Verification items for the finished model (mm, model axes). A direction names the side the tool comes from. Give positions to 0.01 mm unless a question says otherwise; leave off trailing zeros. Loops run counter-clockwise (first coordinate to the right, second up) from the corner with the lowest first, then second, coordinate; pieces in that order, holes last. Notation, with made-up numbers: (11.25, 66) - (66.25, 66) arc R21 ccw to (66.25, 80) - close; hole circle Ø3 at (-17, 37). An arc over 180 degrees is marked (long way). Answer in a Markdown table with one row per item.
Autodesk Fusion 360 part; units mm, degrees
sketch "Sketch1" plane through (0, 0, 0) normal (0, 0, 1) x (1, 0, 0)
  line L0 (-3.85, 0) -> (3.85, 0) construction
  line L1 (-3.85, 0) -> (-8.35, 0) construction
  line L2 (3.85, 0) -> (8.35, 0) construction
  line L3 (0, 0) -> (0, -3.2) construction
  line L4 (-3.85, -4.5) -> (3.85, -4.5)
  line L5 (3.85, 4.5) -> (-3.85, 4.5)
  arc A0 (-3.85, 4.5) -> (-3.85, -4.5) centre (-3.85, 0) ccw
  arc A1 (3.85, -4.5) -> (3.85, 4.5) centre (3.85, 0) ccw
  line L6 (-0.9465, -2.8772) -> (-1.5, -4.5)
  line L7 (0.9465, -2.8772) -> (1.5, -4.5)
  arc A2 (0.9465, -2.8772) -> (-0.9465, -2.8772) centre (0, -3.2) ccw
  line L8 (11.5, -6) -> (-11.5, -6)
  line L9 (-11.5, -6) -> (-11.5, 6)
  line L10 (-11.5, 6) -> (11.5, 6)
  line L11 (11.5, 6) -> (11.5, -6)
  line L12 (11.5, -6) -> (-11.5, 6) construction
  line L13 (-11.5, -6) -> (11.5, 6) construction
  line L14 (-1.15, 2.75) -> (1.15, 2.75)
  line L15 (1.15, -0.75) -> (-1.15, -0.75)
  arc A3 (1.15, -0.75) -> (1.15, 2.75) centre (1.15, 1) ccw
  arc A4 (-1.15, 2.75) -> (-1.15, -0.75) centre (-1.15, 1) ccw
  line L16 (-1.15, 1) -> (1.15, 1)
  dimension "d1" = 9
  dimension "d2" = 16.7
  dimension "d3" = 2
  dimension "d4" = 3.2
  dimension "d5" = 3
  dimension "d6" = 12
  dimension "d7" = 23
  dimension "d12" = 3.5
  dimension "d13" = 2.3
  dimension "d20" = 1
extrude "Extrude1" add sketch "Sketch1" against normal blind 2 contours L4 L5 A0 A1 L6 L7 A2 | L4 L6 L7 A2 | L8 L9 L10 L11 | L14 L15 A3 A4
extrude "Extrude2" add sketch "Sketch1" along normal blind 2 contours L4 L5 A0 A1 L6 L7 A2 | L14 L15 A3 A4
extrude "Extrude3" cut sketch "Sketch1" along normal up to surface (2 mm away) and the other way up to surface (2 mm away) contours L14 L15 A3 A4
fillet "Fillet1" radius 1.5 4 edges at (11.5, -6, -1) (-11.5, -6, -1) (-11.5, 6, -1) (11.5, 6, -1)
equation "d6 = 9 mm + 3 mm"
equation "d13 = 5.8 mm - 3.5 mm"
Q1. Tool access check on faces 5 (the face through (0, -3, 0)), 6 (the face through (3, -4.5, 1)), 7 (the face through (0, -0.75, 0)), 8 (the face through (-8.35, -0.1, 0.99)), 9 (the face through (0, -2.2, 1)). Record the directions out of +Z, -Z, +X, -X, +Y, -Y that give a thin tool (end or side, any length) a straight path to the whole face; none if there is none.
Completed:
| item | result |
|---|---|
| face 5 | +Z |
| face 6 | +Z, +X, -X, -Y |
| face 7 | +Z, -Z |
| face 8 | +Z, -X |
| face 9 | +Z, -Y |
Q2. Sectioned sample at A-A (z = -0.9). Record the cut outline in (x, y), and give its area (3 significant figures).
Completed:
| item | result |
|---|---|
| outline | (-11.5, -4.5) arc R1.5 ccw to (-10, -6) - (10, -6) arc R1.5 ccw to (11.5, -4.5) - (11.5, 4.5) arc R1.5 ccw to (10, 6) - (-10, 6) arc R1.5 ccw to (-11.5, 4.5) - close; hole (-1.15, -0.75) - (1.15, -0.75) arc R1.75 ccw to (1.15, 2.75) - (-1.15, 2.75) arc R1.75 ccw to start |
| area | 256 mm^2 |
Q3. Thickness scan on line 1 (X direction, y = 1, z = -1.05); line 2 (Z direction, x = 0.5, y = -4.5); line 3 (Y direction, x = 0, z = 1.1). Record the ranges inside material, lowest first.
Completed:
| item | result |
|---|---|
| line 1 | -11.5 to -2.9, 2.9 to 11.5 |
| line 2 | -2 to 0 |
| line 3 | -2.2 to -0.75, 2.75 to 4.5 |
Q4. Sectioned sample at B-B (y = 0.5). Record the cut outline in (x, z).
Completed:
| item | result |
|---|---|
| outline | (-11.5, -2) - (-2.83, -2) - (-2.83, 2) - (-8.32, 2) - (-8.32, 0) - (-11.5, 0) - close; (2.83, -2) - (11.5, -2) - (11.5, 0) - (8.32, 0) - (8.32, 2) - (2.83, 2) - close |
Q5. Go/stop test with flat-tipped pins: P1, Ø3, axis at x = 0.5, y = 1.5, coming from the -Z side; P2, Ø0.6, axis at x = 2.5, z = 1.5, coming from the -Y side; P3, Ø1, axis at x = -1.5, z = 1, coming from the +Y side; P4, Ø1.5, axis at y = -0.5, z = 1, coming from the +X side. Record where each tip stops, or that it passes through.
Completed:
| item | result |
|---|---|
| P1 | z = -2 |
| P2 | y = -4.5 |
| P3 | y = 4.5 |
| P4 | x = 8.35 |
Q6. Draft check along Y on faces 1 (the face through (0, 6, -1)), 2 (the face through (0, -1, -2)), 3 (the face through (2.9, 1, 0)), 4 (the face through (0, -6, -1)). Enter one of: +Y half, -Y half, draft (parallel to the pull), parting line (faces both ways), or undercut.
Completed:
| item | result |
|---|---|
| face 1 | +Y half |
| face 2 | draft |
| face 3 | undercut |
| face 4 | -Y half |
Q7. Sectioned sample at C-C (x = -2). Record the cut outline in (y, z), and give its area (3 significant figures).
Completed:
| item | result |
|---|---|
| outline | (-6, -2) - (-0.53, -2) - (-0.53, 2) - (-4.5, 2) - (-4.5, 0) - (-6, 0) - close; (2.53, -2) - (6, -2) - (6, 0) - (4.5, 0) - (4.5, 2) - (2.53, 2) - close |
| area | 29.8 mm^2 |
Q8. Sectioned sample at D-D (y = -4). Record the cut outline in (x, z).
Completed:
| item | result |
|---|---|
| outline | (-11.5, -2) - (11.5, -2) - (11.5, 0) - (5.91, 0) - (5.91, 2) - (1.33, 2) - (1.33, 0) - (-1.33, 0) - (-1.33, 2) - (-5.91, 2) - (-5.91, 0) - (-11.5, 0) - close |
